CAD build for the part. Positions are in the model's coordinates, mm. Face numbers are marked on the shaded views. A direction names the side the tool comes from. Coordinates: 2 decimals unless noted, no trailing zeros. Loops run counter-clockwise (first coordinate to the right, second up) from the corner with the lowest first, then second, coordinate; pieces in that order, holes last. Notation, with made-up numbers: (-36.5, 30) -> (14.5, 30) arc R19 ccw to (14.5, 39) -> close; hole circle Ø8 at (-13, 35.5). An arc over 180 degrees is marked (long way). Answer as CSV lines item,"result". Start each with the question number.
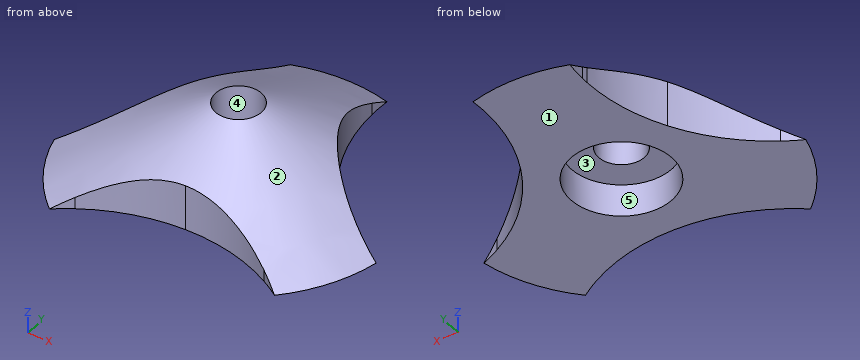
```python
from build123d import *

# Parameters (mm, degrees)
F3_DEPTH       = 25
F4_D           = 10
F4_CBORE_D     = 22
F4_CBORE_DEPTH = 7


with BuildPart() as f1:
    # F0 (on Front) → F1 (revolve)
    with BuildSketch(Plane.XZ):
        Polygon((-35, 0), (0, 0), (0, 20), align=None)
    revolve(axis=Axis((0, 0, 10), (0, 0, -1)))

    # F2 (on Top) → F3 (cut)
    with BuildSketch(Plane.XY):
        with BuildLine():
            Line((2.0660725, -57.6980474345), (20.8136189308, -22.3635104654))
            ThreePointArc((20.8136189308, -22.3635104654), (11.0295606596, -18.7152835508), (0.6346554831, -17.7236675729))
            Line((0.6346554831, -17.7236675729), (2.0660725, -57.6980474345))
        make_face()
        with BuildLine():
            ThreePointArc((-19.1607609308, -23.7949274822), (-17.310803703, -92.6914277888), (42.0660725, -57.6980474345))
            ThreePointArc((42.0660725, -57.6980474345), (36.3436297148, -37.0813291849), (20.8136189308, -22.3635104654))
            Line((20.8136189308, -22.3635104654), (2.0660725, -57.6980474345))
            Line((2.0660725, -57.6980474345), (-19.1607609308, -23.7949274822))
        make_face()
        with BuildLine():
            ThreePointArc((0.6346554831, -17.7236675729), (-9.6627009891, -19.4562395217), (-19.1607609308, -23.7949274822))
            Line((-19.1607609308, -23.7949274822), (2.0660725, -57.6980474345))
            Line((2.0660725, -57.6980474345), (0.6346554831, -17.7236675729))
        make_face()
        with BuildLine():
            Line((48.9349385771, 30.6382949883), (30.1873921462, -4.6962419808))
            ThreePointArc((30.1873921462, -4.6962419808), (69.5516568267, -3.6392622266), (88.9349385771, 30.6382949883))
            ThreePointArc((88.9349385771, 30.6382949883), (48.2191154377, 70.6318894408), (8.9605587154, 29.2068779715))
            Line((8.9605587154, 29.2068779715), (48.9349385771, 30.6382949883))
        make_face()
        with BuildLine():
            ThreePointArc((8.9605587154, 29.2068779715), (10.6931306643, 18.9095214992), (15.0318186248, 9.4114615575))
            Line((15.0318186248, 9.4114615575), (48.9349385771, 30.6382949883))
            Line((48.9349385771, 30.6382949883), (8.9605587154, 29.2068779715))
        make_face()
        with BuildLine():
            ThreePointArc((15.0318186248, 9.4114615575), (21.6809481825, 1.3599752351), (30.1873921462, -4.6962419808))
            Line((30.1873921462, -4.6962419808), (48.9349385771, 30.6382949883))
            Line((48.9349385771, 30.6382949883), (15.0318186248, 9.4114615575))
        make_face()
        with BuildLine():
            ThreePointArc((-11.0266312154, 28.4911694631), (-86.3355480462, 45.8072988771), (-29.7741776462, -6.8433675061))
            Line((-29.7741776462, -6.8433675061), (-51.001011077, 27.0597524462))
            Line((-51.001011077, 27.0597524462), (-11.0266312154, 28.4911694631))
        make_face()
        with BuildLine():
            ThreePointArc((-11.001011077, 27.0597524462), (-11.0074166245, 27.7755755856), (-11.0266312154, 28.4911694631))
            Line((-11.0266312154, 28.4911694631), (-51.001011077, 27.0597524462))
            Line((-51.001011077, 27.0597524462), (-15.6664741079, 8.3122060154))
            ThreePointArc((-15.6664741079, 8.3122060154), (-12.1848966478, 17.4000805772), (-11.001011077, 27.0597524462))
        make_face()
        with BuildLine():
            Line((-51.001011077, 27.0597524462), (-29.7741776462, -6.8433675061))
            ThreePointArc((-29.7741776462, -6.8433675061), (-21.7226913238, -0.1942379484), (-15.6664741079, 8.3122060154))
            Line((-15.6664741079, 8.3122060154), (-51.001011077, 27.0597524462))
        make_face()
    extrude(amount=F3_DEPTH, mode=Mode.SUBTRACT)

    # F4 (through all)
    with Locations(Plane(origin=(0, 0, 0), x_dir=(1, 0, 0), z_dir=(0, 0, -1))):
        with Locations((0, 0)):
            CounterBoreHole(F4_D / 2, F4_CBORE_D / 2, F4_CBORE_DEPTH)


solid = f1.part
```
Q1. Saw through at A-A (y = 0). List the corners of the cut face in (x, z).
Q2. Saw through at C-C (z = 15). List the corners of the cut face in (x, y).
Q3. Which spindle directions (+Z, -Z, +X, -X, +Y, -Y) get a long thin tool onto all of the face, cutting with end or side? Do the marked faces 4 and 5. Say none if no direction does.
Q4. Two-plate mould, pull along X, no slides. Class the marked faces 1, 2 and 3: pulls with the +X half, pulls with the -X half, needs draft (parallel to the pull), parting line crosses it, or undercut.
Q5. Saw through at B-B (z = 5). List the corners of the cut face in (x, y).
Q6. Probe probe 1 along Y at (x, z) = (0, 2.25); probe 2 along Y at (x, z) = (-5.5, 6.25); probe 3 along X at (y, z) = (2.5, 5.25). List the from-to ranges inside material, lowest first. Write a range as from..to.
Q7. Pin check, flat tips, straight feed: pin 1 Ø17.5 at (x, y) = (0, 0) entering from +Z; pin 2 Ø3 at (x, y) = (3, 11) entering from +Z; pin 3 Ø3 at (x, y) = (3, -17) entering from +Z; pin 4 Ø3 at (y, z) = (-10.5, 3.5) entering from -X. Stop position of each tip, or through.
Ans:
1,outline,"(-21.54, 0) -> (-11, 0) -> (-11, 7) -> (-5, 7) -> (-5, 17.14) -> (-21.54, 7.69) -> close; (5, 7) -> (11, 7) -> (11, 0) -> (23.22, 0) -> (23.22, 6.73) -> (5, 17.14) -> close"
2,outline,"circle Ø17.5 at (0, 0); hole circle Ø10 at (0, 0)"
3,face 4,"+Z, -Z"
3,face 5,"-Z"
4,face 1,"needs draft"
4,face 2,"parting line crosses it"
4,face 3,"undercut"
5,outline,"(-25.93, -4.11) arc R26.25 ccw to (-15.02, -21.53) arc R40 cw to (16.52, -20.4) arc R26.25 ccw to (26.15, -2.24) arc R40 cw to (9.41, 24.51) arc R26.25 ccw to (-11.14, 23.77) arc R40 cw to start; hole circle Ø22 at (0, 0)"
6,probe 1,"y = -17.75..-11, 11..31.06"
6,probe 2,"y = -18.42..-9.53, 9.53..23.43"
6,probe 3,"x = -19.43..-10.71, 10.71..20.51"
7,pin 1,"stops at z = 17.14"
7,pin 2,"stops at z = 14.34"
7,pin 3,"stops at z = 10.99"
7,pin 4,"stops at x = -29.75"
